Can you work these out from the drawing? Everything is in mm from the part's minimum corner. Coordinates: 2 decimals unless noted, no trailing zeros. Loops run counter-clockwise (first coordinate to the right, second up) from the corner with the lowest first, then second, coordinate; pieces in that order, holes last. Notation, with made-up numbers: M 71,86 L 128,86 A15 cw 128,115 Z; hole C 89.25,69.25 d3. An arc over 180 degrees is marked long. Write each question's results on one line, items separated by ' | '.
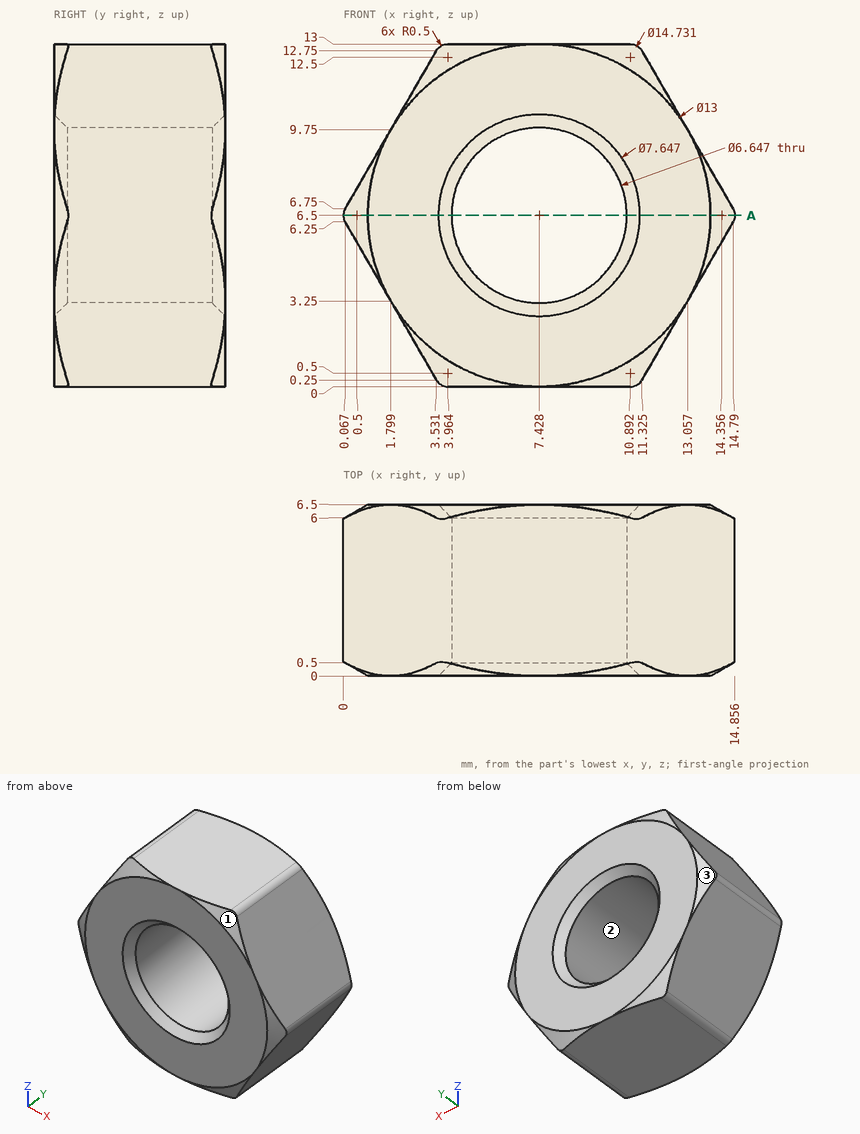
(1) If we mould it in two halves opening along X, with no side actions, what happens to the marked faces 1, 2 and 3? For each: released by +X, released by -X, zero draft, split by the parting line, or undercut.
Reported:
face 1: released by +X | face 2: undercut | face 3: released by -X
(2) Please list where these lines run through material, in increasing order: probe 1 along Z at (x, y) = (7.5, 5.25); probe 2 along X at (y, z) = (2.45, 6.5) (1 decimal); probe 3 along Z at (x, y) = (8.5, 0.75) (1 decimal). Write a range as from..to.
Reported:
probe 1: z = 0..3.18, 9.82..13 | probe 2: x = 0..4.1, 10.8..14.9 | probe 3: z = 0..3.4, 9.6..13
(3) Will these pins go through, and if not, where does the flat tip stop? P1, Ø5, axis at x = 10, z = 5.5, coming from the +Y side; P2, Ø1.5, axis at y = 5, z = 10.5, coming from the -X side.
Reported:
P1: stops at y = 6.5 | P2: stops at x = 1.8
(4) Imagine slicing it at A-A, the plane z = 6.5. List the corners of the cut face in (x, y) for me (1 decimal).
Reported:
outline: M 0,0.5 L 0.9,0 L 3.6,0 L 4.1,0.5 L 4.1,6 L 3.6,6.5 L 0.9,6.5 L 0,6 Z; M 10.8,0.5 L 11.3,0 L 13.9,0 L 14.9,0.5 L 14.9,6 L 13.9,6.5 L 11.3,6.5 L 10.8,6 Z
